```python
from build123d import *

# Parameters (mm, degrees)
BOSS_EXTRUDE1_DEPTH      = 6.35
F_5_16_18_TAPPED_HOLE1_D = 6.5278
CUT_EXTRUDE1_START       = -0.25
CUT_EXTRUDE1_DEPTH       = 0.25
CUT_EXTRUDE5_DEPTH       = 13.45
CUT_EXTRUDE6_DEPTH       = 5.00000016
CUT_EXTRUDE3_DEPTH       = 2.5
CUT_EXTRUDE4_DEPTH       = 10.95
CHAMFER1_SIZE            = 4.7625


with BuildPart() as part:
    # Sketch1 → Boss-Extrude1 (new body, symmetric)
    with BuildSketch(Plane(origin=(0, 0, 0), x_dir=(1, 0, 0), z_dir=(0, 1, 0))):
        Polygon((-33.3375, 57.15), (-58.7375, 57.15), (-58.7375, 19.05), (-33.3375, -6.35), (-33.3375, -57.15), (33.3375, -57.15), (33.3375, -6.35), (58.7375, 19.05), (58.7375, 57.15), (33.3375, 57.15), align=None)
    extrude(amount=BOSS_EXTRUDE1_DEPTH, both=True)

    # 5/16-18 Tapped Hole1 (through all)
    with Locations(Plane(origin=(0, 6.35, 0), x_dir=(1, 0, 0), z_dir=(0, 1, 0))):
        with Locations((-44.45, 38.1), (44.45, 38.1)):
            Hole(F_5_16_18_TAPPED_HOLE1_D / 2)

    # Sketch4 → Cut-Extrude1 (cut)
    with BuildSketch(Plane(origin=(0, 6.35, 0), x_dir=(1, 0, 0), z_dir=(0, 1, 0)).offset(CUT_EXTRUDE1_START)):
        Polygon((33.3375, -57.15), (33.3375, -6.35), (58.7375, 19.05), (58.7375, 57.15), (-58.7375, 57.15), (-58.7375, 19.05), (-33.3375, -6.35), (-33.3375, -57.15), align=None)
    extrude(amount=CUT_EXTRUDE1_DEPTH, mode=Mode.SUBTRACT)

    # Sketch12 → Cut-Extrude5 (cut, through all)
    with BuildSketch(Plane.XZ.offset(6.35)):
        with BuildLine():
            Line((26.324, -4.92), (26.324, -11.27))
            ThreePointArc((26.324, -11.27), (23.57, -14.024), (20.816, -11.27))
            Line((20.816, -11.27), (20.816, -4.92))
            ThreePointArc((20.816, -4.92), (23.57, -2.166), (26.324, -4.92))
        make_face()
        with BuildLine():
            Line((20.816, 35.87), (20.816, 42.22))
            ThreePointArc((20.816, 42.22), (23.57, 44.974), (26.324, 42.22))
            Line((26.324, 42.22), (26.324, 35.87))
            ThreePointArc((26.324, 35.87), (23.57, 33.116), (20.816, 35.87))
        make_face()
    cut_extrude5 = extrude(amount=-CUT_EXTRUDE5_DEPTH, mode=Mode.SUBTRACT)

    # Sketch13 → Cut-Extrude6 (cut)
    with BuildSketch(Plane.XZ.offset(6.35)):
        with BuildLine():
            Line((19.069999983, -15.945999919), (19.069999983, -0.244000081))
            ThreePointArc((19.069999983, -0.244000081), (23.57, 4.255999936), (28.070000017, -0.244000081))
            Line((28.070000017, -0.244000081), (28.070000017, -15.945999919))
            ThreePointArc((28.070000017, -15.945999919), (23.57, -20.445999936), (19.069999983, -15.945999919))
        make_face()
        with BuildLine():
            Line((19.069999983, 31.194000081), (19.069999983, 46.895999919))
            ThreePointArc((19.069999983, 46.895999919), (23.57, 51.395999936), (28.070000017, 46.895999919))
            Line((28.070000017, 46.895999919), (28.070000017, 31.194000081))
            ThreePointArc((28.070000017, 31.194000081), (23.57, 26.694000064), (19.069999983, 31.194000081))
        make_face()
    cut_extrude6 = extrude(amount=-CUT_EXTRUDE6_DEPTH, mode=Mode.SUBTRACT)

    # Mirror1: Cut-Extrude5, Cut-Extrude6 across plane
    add(cut_extrude5.mirror(Plane(origin=(0, 0, 0), x_dir=(0, 0, 1), z_dir=(1, 0, 0))), mode=Mode.SUBTRACT)
    add(cut_extrude6.mirror(Plane(origin=(0, 0, 0), x_dir=(0, 0, 1), z_dir=(1, 0, 0))), mode=Mode.SUBTRACT)

    # Sketch8 → Cut-Extrude3 (cut)
    with BuildSketch(Plane(origin=(0, 6.1, 0), x_dir=(1, 0, 0), z_dir=(0, 1, 0))):
        with BuildLine():
            Line((-22.175, -18.65), (-22.175, -12.3))
            ThreePointArc((-22.175, -12.3), (0, 9.875), (22.175, -12.3))
            Line((22.175, -12.3), (22.175, -18.65))
            ThreePointArc((22.175, -18.65), (0, -40.825), (-22.175, -18.65))
        make_face()
    extrude(amount=-CUT_EXTRUDE3_DEPTH, mode=Mode.SUBTRACT)

    # Sketch9 → Cut-Extrude4 (cut, through all)
    with BuildSketch(Plane(origin=(0, 3.6, 0), x_dir=(1, 0, 0), z_dir=(0, 1, 0))):
        with BuildLine():
            Line((-15.875, -18.65), (-15.875, -12.3))
            ThreePointArc((-15.875, -12.3), (0, 3.575), (15.875, -12.3))
            Line((15.875, -12.3), (15.875, -18.65))
            ThreePointArc((15.875, -18.65), (0, -34.525), (-15.875, -18.65))
        make_face()
    extrude(amount=-CUT_EXTRUDE4_DEPTH, mode=Mode.SUBTRACT)

    # Chamfer1
    chamfer1_edges = [part.edges().sort_by_distance(p)[0] for p in [
        (33.3375, -0.125, 57.15),
        (-33.3375, -0.125, 57.15),
        (-58.7375, -0.125, -57.15),
        (58.7375, -0.125, -57.15),
    ]]
    chamfer(chamfer1_edges, length=CHAMFER1_SIZE)


solid = part.part
```
Verification items for the finished model (mm, model axes). A direction names the side the tool comes from. Coordinates: 2 decimals unless noted, no trailing zeros. Order: outer loops, then holes, each group sorted by start corner. A loop starts at its lowest first (then second) coordinate and runs counter-clockwise, first axis right, second up. Notation, with made-up numbers: (0, 7) -> (26, 7) arc R8 ccw to (26, 21) -> close; hole circle Ø8 at (23.5, 30). An arc over 180 degrees is marked (long way). Put each result on its own line as item: value. Start each with the question number.
1) Cross-section at C-C (z = -8). Enter the section's corners in (x, y), plus the area to 3 significant figures.
2) Release check for a two-part mould opening along Z. For faces 1 (the cylindrical face through (-23.471, -3.885, 51.395)), 2 (the flat face through (58.738, 0, -35)), 3 (the flat face through (-56.323, -0.038, -54.802)), 4 (the flat face through (45.86, -0.04, -6.17)) record: pulls with the +Z half, pulls with the -Z half, needs draft (parallel to the pull), parting line crosses it, or undercut.
3) Cross-section at D-D (x = 23.57). Enter the section's corners in (y, z), plus the area to 3 significant figures.
4) Tool access check on faces 5 (the cylindrical face through (-23.509, 2.323, -2.167)), 6 (the cylindrical face through (-23.669, -3.885, 26.695)). Record the directions out of +Z, -Z, +X, -X, +Y, -Y that give a thin tool (end or side, any length) a straight path to the whole face; none if there is none.
5) Material ranges on L1, parallel to X at y = 3.75, z = -38.1; L2, parallel to X at y = 5, z = -13; L3, parallel to X at y = 4, z = 34, recorded low to high.
6) Go/stop test with flat-tipped pins: pin 1 (7 mm diameter, centred on y = 4, z = 38, fed in from +X); pin 2 (2.5 mm diameter, centred on y = -5, z = -10, fed in from +X); pin 3 (2 mm diameter, centred on y = -2, z = -3.5, fed in from +X). Record where each tip stops, or that it passes through.
7) Cross-section at A-A (x = 0). Enter the section's corners in (y, z) (3 decimals).
8) Cross-section at B-B (y = -4.25). State how many separate pieces and enclosed holes the cut face has, plus the area to 3 significant figures.
Geometry check:
1. outline: (-47.69, -6.35) -> (-28.07, -6.35) -> (-28.07, -1.35) -> (-26.32, -1.35) -> (-26.32, 6.1) -> (-47.69, 6.1) -> close; (-20.82, -1.35) -> (-19.07, -1.35) -> (-19.07, -6.35) -> (19.07, -6.35) -> (19.07, -1.35) -> (20.82, -1.35) -> (20.82, 6.1) -> (8.92, 6.1) -> (8.92, 3.6) -> (-8.92, 3.6) -> (-8.92, 6.1) -> (-20.82, 6.1) -> close; (26.32, -1.35) -> (28.07, -1.35) -> (28.07, -6.35) -> (47.69, -6.35) -> (47.69, 6.1) -> (26.32, 6.1) -> close
1. area: 971 mm^2
2. face 1: undercut
2. face 2: needs draft
2. face 3: pulls with the -Z half
2. face 4: pulls with the +Z half
3. outline: (-6.35, -57.15) -> (6.1, -57.15) -> (6.1, -14.02) -> (-1.35, -14.02) -> (-1.35, -20.45) -> (-6.35, -20.45) -> close; (-6.35, 4.26) -> (-1.35, 4.26) -> (-1.35, -2.17) -> (6.1, -2.17) -> (6.1, 33.12) -> (-1.35, 33.12) -> (-1.35, 26.69) -> (-6.35, 26.69) -> close; (-6.35, 51.4) -> (-1.35, 51.4) -> (-1.35, 44.97) -> (6.1, 44.97) -> (6.1, 57.15) -> (-6.35, 57.15) -> close
3. area: 999 mm^2
4. face 5: +Y, -Y
4. face 6: -Y
5. L1: x = -58.74 to -47.71, -41.19 to 41.19, 47.71 to 58.74
5. L2: x = -52.69 to -25.71, -21.43 to 21.43, 25.71 to 52.69
5. L3: x = -33.34 to -25.59, -21.55 to -16, 16 to 21.55, 25.59 to 33.34
6. pin 1: stops at x = 33.34
6. pin 2: stops at x = 50.94
6. pin 3: stops at x = 44.19
7. outline: (-6.35, -57.15) -> (6.1, -57.15) -> (6.1, -9.875) -> (3.6, -9.875) -> (3.6, -3.575) -> (-6.35, -3.575) -> close; (-6.35, 34.525) -> (3.6, 34.525) -> (3.6, 40.825) -> (6.1, 40.825) -> (6.1, 57.15) -> (-6.35, 57.15) -> close
8. separate pieces: 1
8. enclosed holes: 7
8. area: 8,280 mm^2
